The model under review builds one solid part; all positions refer to its coordinate system, in mm. A direction names the side the tool comes from. Round coordinates to 2 decimals unless told otherwise and drop trailing zeros. Order: outer loops, then holes, each group sorted by start corner. A loop starts at its lowest first (then second) coordinate and runs counter-clockwise, first axis right, second up.
```python
from build123d import *

# Parameters (mm, degrees)
SKETCH_W        = 220
SKETCH_H        = 300
SKETCH_W_2      = 129
SKETCH_H_2      = 237
PAD_DEPTH       = 3
SKETCH001_W     = 143
SKETCH001_H     = 245
SKETCH001_W_2   = 129
SKETCH001_H_2   = 237
POCKET_DEPTH    = 2
SKETCH002_R     = 7.9
SKETCH002_R_2   = 1
SKETCH002_W     = 3.6
SKETCH002_H     = 10
SKETCH002_W_2   = 35
SKETCH002_H_2   = 3
SKETCH002_W_3   = 15
POCKET001_DEPTH = 3.001
SKETCH003_R     = 3.6
SKETCH003_R_2   = 1
POCKET002_DEPTH = 5


with BuildPart() as part:
    # Sketch → Pad (new body)
    with BuildSketch(Plane.XY):
        with Locations((110, 150)):
            Rectangle(SKETCH_W, SKETCH_H)
        with Locations((110, 133.5)):
            Rectangle(SKETCH_W_2, SKETCH_H_2, mode=Mode.SUBTRACT)
    extrude(amount=PAD_DEPTH)

    # Sketch001 (on Face9 of Pad) → Pocket (cut)
    with BuildSketch(Plane(origin=(0, 0, 0), x_dir=(1, 0, 0), z_dir=(0, 0, -1))):
        with Locations((113, -134.5)):
            Rectangle(SKETCH001_W, SKETCH001_H)
        with Locations((110, -133.5)):
            Rectangle(SKETCH001_W_2, SKETCH001_H_2, mode=Mode.SUBTRACT)
    extrude(amount=-POCKET_DEPTH, mode=Mode.SUBTRACT)

    # Sketch002 (on Face5 of Pocket) → Pocket001 (cut, through all)
    with BuildSketch(Plane.XY.offset(3)):
        with Locations((17.75, 185.5)):
            Circle(SKETCH002_R)
        with Locations((17.75, 160)):
            Circle(SKETCH002_R)
        with Locations((9, 151.5)):
            Circle(SKETCH002_R_2)
        with Locations((26.5, 151.5)):
            Circle(SKETCH002_R_2)
        with Locations((9, 194)):
            Circle(SKETCH002_R_2)
        with Locations((26.5, 194)):
            Circle(SKETCH002_R_2)
        with Locations((202.25, 185.5)):
            Circle(SKETCH002_R)
        with Locations((202.25, 160)):
            Circle(SKETCH002_R)
        with Locations((193.5, 151.5)):
            Circle(SKETCH002_R_2)
        with Locations((211, 151.5)):
            Circle(SKETCH002_R_2)
        with Locations((193.5, 194)):
            Circle(SKETCH002_R_2)
        with Locations((211, 194)):
            Circle(SKETCH002_R_2)
        with Locations((10.4, 172.75)):
            Rectangle(SKETCH002_W, SKETCH002_H)
        with Locations((194.9, 172.75)):
            Rectangle(SKETCH002_W, SKETCH002_H)
        with Locations((42.5, 1.5)):
            Rectangle(SKETCH002_W_2, SKETCH002_H_2)
        with Locations((87.5, 1.5)):
            Rectangle(SKETCH002_W_2, SKETCH002_H_2)
        with Locations((132.5, 1.5)):
            Rectangle(SKETCH002_W_2, SKETCH002_H_2)
        with Locations((177.5, 1.5)):
            Rectangle(SKETCH002_W_2, SKETCH002_H_2)
        with Locations((7.5, 1.5)):
            Rectangle(SKETCH002_W_3, SKETCH002_H_2)
        with Locations((212.5, 1.5)):
            Rectangle(SKETCH002_W_3, SKETCH002_H_2)
    extrude(amount=-POCKET001_DEPTH, mode=Mode.SUBTRACT)

    # Sketch003 (on Face5 of Pocket001) → Pocket002 (cut)
    with BuildSketch(Plane(origin=(15, 0, 0), x_dir=(0, -1, 0), z_dir=(-1, 0, 0))):
        with Locations((110, 272)):
            Circle(SKETCH003_R)
        with Locations((110, 261.5)):
            Circle(SKETCH003_R_2)
        with Locations((110, 282.5)):
            Circle(SKETCH003_R_2)
        with Locations((122.5, 261.5)):
            Circle(SKETCH003_R_2)
        with Locations((122.5, 282.5)):
            Circle(SKETCH003_R_2)
    extrude(amount=-POCKET002_DEPTH, mode=Mode.SUBTRACT)


solid = part.part
```
(1) For faces 1 (the flat face through (35, 185, 3)), 2 (the flat face through (176, 134, 2)), list the 3-axis set-ups (+Z, -Z, +X, -X, +Y, -Y) from which the entire face can be reached by the end or side of a thin tool; tool diameter is ignored.
Data:
face 1: +Z, +X, -X, +Y, -Y
face 2: -Z
(2) Consider section A-A (y = 110.5). Write out the cut boundary in (x, z).
Data:
outline: (0, 0) - (41.5, 0) - (41.5, 2) - (45.5, 2) - (45.5, 3) - (0, 3) - close; (174.5, 2) - (184.5, 2) - (184.5, 0) - (220, 0) - (220, 3) - (174.5, 3) - close
(3) Draft analysis for pull direction Y (two halves, no side actions). For faces 3 (the cylindrical face through (9.858, 160.347, 1.521)), 4 (the flat face through (35, 185, 0)), state which applies: pulls with the +Y half, pulls with the -Y half, needs draft (parallel to the pull), parting line crosses it, or undercut.
Data:
face 3: undercut
face 4: needs draft
(4) To check wall thickness, follow probe 1 along X at (y, z) = (151.5, 1.8); probe 2 along Y at (x, z) = (202.25, 2.2); probe 3 along X at (y, z) = (171, 0.35). State the ranges of each line that lie inside material, in increasing order.
Data:
probe 1: x = 0 to 8, 10 to 25.5, 27.5 to 41.5, 184.5 to 192.5, 194.5 to 210, 212 to 220
probe 2: y = 0 to 152.1, 167.9 to 177.6, 193.4 to 300
probe 3: x = 0 to 8.6, 12.2 to 41.5, 184.5 to 193.1, 196.7 to 220
(5) Insertion check: pin 1 (0.9 mm diameter, centred on x = 194.5, z = 1, fed in from -Y); pin 2 (8 mm diameter, centred on x = 130, y = 251, fed in from -Z). Each pin has a flat end and moves straight along its axis. Give the tip position at first contact, or say it passes through.
Data:
pin 1: stops at y = 3
pin 2: stops at z = 2
(6) Consider section B-B (x = 145). Write out the cut boundary in (y, z).
Data:
outline: (3, 0) - (12, 0) - (12, 2) - (15, 2) - (15, 3) - (3, 3) - close; (252, 2) - (257, 2) - (257, 0) - (300, 0) - (300, 3) - (252, 3) - close
(7) Consider section C-C (y = 160). Write out the cut boundary in (x, z), and give its area (3 significant figures).
Data:
outline: (0, 0) - (9.85, 0) - (9.85, 3) - (0, 3) - close; (25.65, 0) - (41.5, 0) - (41.5, 2) - (45.5, 2) - (45.5, 3) - (25.65, 3) - close; (174.5, 2) - (184.5, 2) - (184.5, 0) - (194.35, 0) - (194.35, 3) - (174.5, 3) - close; (210.15, 0) - (220, 0) - (220, 3) - (210.15, 3) - close
area: 150 mm2
